```python
from build123d import *

# Parameters (mm, degrees)
F1_DEPTH = 25.4
F2_R     = 2.54
F3_R     = 4.7625
F4_DEPTH = 152.4


with BuildPart() as f1:
    # F0 (on Front) → F1 (new body)
    with BuildSketch(Plane.XZ):
        Polygon((-69.85, -56.106601), (0, -56.106601), (69.85, -56.106601), (69.85, -52.931601), (69.85, 23.268399), (66.675, 23.268399), (66.675, -52.931601), (-66.675, -52.931601), (-66.675, 23.268399), (-69.85, 23.268399), (-69.85, -52.931601), align=None)
    extrude(amount=F1_DEPTH)

    # F2
    f2_edges = [f1.edges().sort_by_distance(p)[0] for p in [
        (-69.85, -12.7, -56.106601),
        (69.85, -12.7, -56.106601),
    ]]
    fillet(f2_edges, radius=F2_R)

    # F3 (on face) → F4 (cut)
    with BuildSketch(Plane(origin=(-69.85, 0, 0), x_dir=(0, -1, 0), z_dir=(-1, 0, 0))):
        with Locations((12.7, 4.218399)):
            Circle(F3_R)
    extrude(amount=-F4_DEPTH, mode=Mode.SUBTRACT)


solid = f1.part
```
Source: CAD feature listing. Evaluate the final solid. Frame: model axes, mm. A direction names the side the tool comes from. Round coordinates to 2 decimals unless told otherwise and drop trailing zeros. Write each loop counter-clockwise with the first axis right and the second up, starting at its lowest first coordinate (ties: lowest second). Pieces come first, ordered by that corner, then holes. Notation, with made-up numbers: M 47,50 L 100,50 A30 cw 100,85 Z; hole C -30.5,-1.75 d3. An arc over 180 degrees is marked long. Use CSV: the item, a comma, the result in double quotes. Start each with the question number.
Q1. Cut plane A-A on z = -25.5. Output: boundary loops of the cut face in (x, y) (3 decimals).
Q2. Line query: line 1 (X direction, y = -16.75, z = -23) (3 decimals); line 2 (Z direction, x = 68.2, y = -12.7); line 3 (Z direction, x = 39, y = -14.75). Output: solid intervals per line, ascending. Write a range as from..to.
Q3. Pull-direction query (Z, two-part tool) for faces 1 (the face through (-68.285, -7.942, 4.428)), 2 (the face through (-66.675, -13, -15)), 3 (the face through (1, -13, -52.932)); classes: +Z half, -Z half, draft (parallel to the pull), parting line (faces both ways), or undercut.
Q4. Cut plane D-D on x = 28.5. Output: boundary loops of the cut face in (y, z).
Q5. Cut plane C-C on y = -22.25. Output: boundary loops of the cut face in (x, z) (3 decimals), plus the area to 3 significant figures.
Q6. Access query for faces 4 (the face through (-1, -13, -56.107)), 5 (the face through (66.675, -13, -14)). Directions: +Z, -Z, +X, -X, +Y, -Y. A direction counts if a zero-diameter tool reaches every point of the face in a straight line with its end or side. Return the directions, or none.
Q7. Cut plane B-B on y = -12.7. Output: boundary loops of the cut face in (x, z) (3 decimals), plus the area to 3 significant figures.
Results found:
1,outline,"M -69.85,-25.4 L -66.675,-25.4 L -66.675,0 L -69.85,0 Z; M 66.675,-25.4 L 69.85,-25.4 L 69.85,0 L 66.675,0 Z"
2,line 1,"-69.85..-66.675, 66.675..69.85"
2,line 2,"-55.95..-0.54, 8.98..23.27"
2,line 3,"-56.11..-52.93"
3,face 1,"undercut"
3,face 2,"draft"
3,face 3,"+Z half"
4,outline,"M -25.4,-56.11 L 0,-56.11 L 0,-52.93 L -25.4,-52.93 Z"
5,outline,"M -69.85,-53.567 A2.54 ccw -67.31,-56.107 L 67.31,-56.107 A2.54 ccw 69.85,-53.567 L 69.85,23.268 L 66.675,23.268 L 66.675,-52.932 L -66.675,-52.932 L -66.675,23.268 L -69.85,23.268 Z"
5,area,"925 mm^2"
6,face 4,"-Z, +X, -X, +Y, -Y"
6,face 5,"+Z, +Y, -Y"
7,outline,"M -69.85,-53.567 A2.54 ccw -67.31,-56.107 L 67.31,-56.107 A2.54 ccw 69.85,-53.567 L 69.85,-0.544 L 66.675,-0.544 L 66.675,-52.932 L -66.675,-52.932 L -66.675,-0.544 L -69.85,-0.544 Z; M -69.85,8.981 L -66.675,8.981 L -66.675,23.268 L -69.85,23.268 Z; M 66.675,8.981 L 69.85,8.981 L 69.85,23.268 L 66.675,23.268 Z"
7,area,"864 mm^2"
